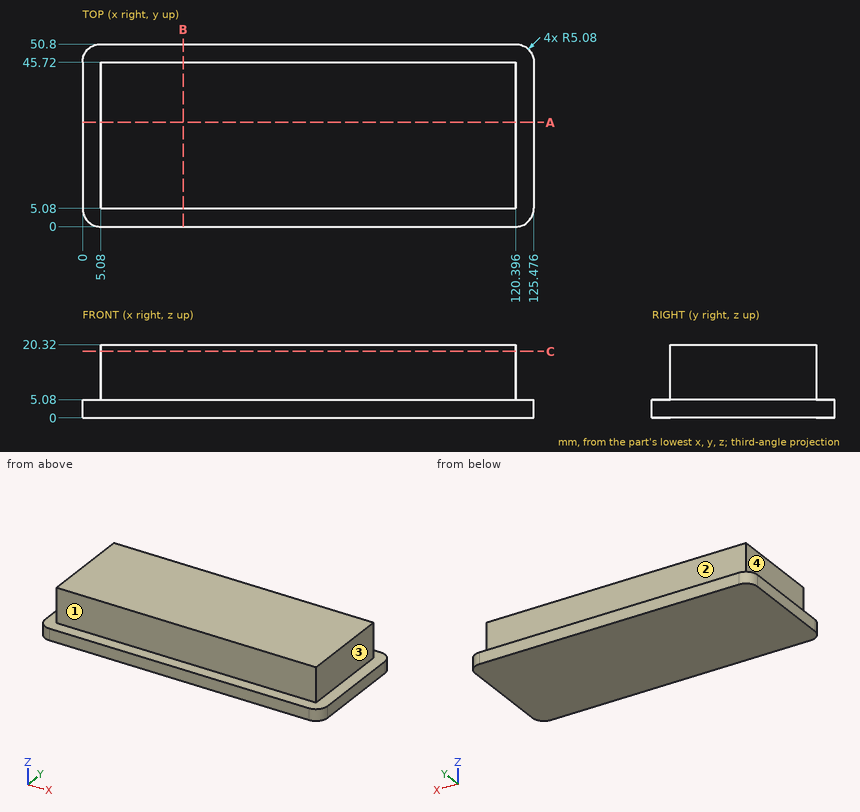
Source: three-view drawing plus pictorial views. Frame: mm from the lowest corner of the part. A direction names the side the tool comes from. Give positions to 0.01 mm unless a question says otherwise; leave off trailing zeros. Order: outer loops, then holes, each group sorted by start corner. A loop starts at its lowest first (then second) coordinate and runs counter-clockwise, first axis right, second up. Notation, with made-up numbers: (40, 84.25) - (54, 84.25) arc R11 ccw to (54, 100.25) - close; hole circle Ø4 at (54.5, 25.5). An arc over 180 degrees is marked (long way). Answer as a JSON object with one key per item and string values. Group by question number.
Q1. Cut plane B-B, the plane x = 28. Output: boundary loops of the cut face in (y, z).
Q2. Cut plane A-A, the plane y = 29. Output: boundary loops of the cut face in (x, z), then the cut area to 3 significant figures.
Q3. First-contact query: pin 1 Ø4.5 at (y, z) = (25.5, 13.5) entering from +X; pin 2 Ø12 at (x, z) = (31.5, 2) entering from -Y; pin 3 Ø4.5 at (y, z) = (29.5, 14) entering from -X; pin 4 Ø7.5 at (x, z) = (52.5, 15.5) entering from +Y. Flat tips, straight axial feed; report the tip coordinate or a pass-through.
Q4. Line query: probe 1 along Y at (x, z) = (74, 13); probe 2 along X at (y, z) = (38, 17.5); probe 3 along Z at (x, y) = (39, 49.5). Output: solid intervals per line, ascending.
Q5. Set-up query: the marked faces 1, 2, 3 and 4. Return all of +Z, -Z, +X, -X, +Y, -Y with unobstructed straight access to the full face (end or side cutting, diameter ignored); none if empty.
Q6. Cut plane C-C, the plane z = 18.5. Output: boundary loops of the cut face in (x, y), then the cut area to 3 significant figures.
Results:
{
 "1": {"outline": "(0, 0) - (50.8, 0) - (50.8, 5.08) - (45.72, 5.08) - (45.72, 20.32) - (5.08, 20.32) - (5.08, 5.08) - (0, 5.08) - close"},
 "2": {"outline": "(0, 0) - (125.48, 0) - (125.48, 5.08) - (120.4, 5.08) - (120.4, 20.32) - (5.08, 20.32) - (5.08, 5.08) - (0, 5.08) - close", "area": "2,390 mm^2"},
 "3": {"pin 1": "x = 120.4", "pin 2": "y = 0", "pin 3": "x = 5.08", "pin 4": "y = 45.72"},
 "4": {"probe 1": "5.08 to 45.72", "probe 2": "5.08 to 120.4", "probe 3": "0 to 5.08"},
 "5": {"face 1": "+Z, +X, -X, -Y", "face 2": "+Z, +X, -X, +Y", "face 3": "+Z, +X, +Y, -Y", "face 4": "+Z, -X, +Y, -Y"},
 "6": {"outline": "(5.08, 5.08) - (120.4, 5.08) - (120.4, 45.72) - (5.08, 45.72) - close", "area": "4,690 mm^2"}
}
